Geometry: final body of the model. Coordinates: model frame, mm. Face numbers are marked on the shaded views. A direction names the side the tool comes from. Give positions to 0.01 mm unless a question says otherwise; leave off trailing zeros. Loops run counter-clockwise (first coordinate to the right, second up) from the corner with the lowest first, then second, coordinate; pieces in that order, holes last.
1. Section D-D, the plane y = -3.75. Output: boundary loops of the cut face in (x, z).
2. Material intervals for line 1 along Y through (x, z) = (12, -2.75); line 2 along Z through (x, y) = (28, -2); line 3 along Z through (x, y) = (35.5, 1.5), sorted ascending.
3. Section A-A, the plane z = 0. Output: boundary loops of the cut face in (x, y) (3 decimals).
4. Access query for the marked faces 1 and 2. Directions: +Z, -Z, +X, -X, +Y, -Y. A direction counts if a zero-diameter tool reaches every point of the face in a straight line with its end or side. Return the directions, or none.
5. First-contact query: P1, Ø2, axis at x = 21, z = -3.5, coming from the -Y side; P2, Ø1.5, axis at y = 3.5, z = 3.5, coming from the -X side; P3, Ø2, axis at y = -1, z = -3.5, coming from the +X side. Flat tips, straight axial feed; report the tip coordinate or a pass-through.
6. Section C-C, the plane x = 26. Output: boundary loops of the cut face in (y, z) (3 decimals).
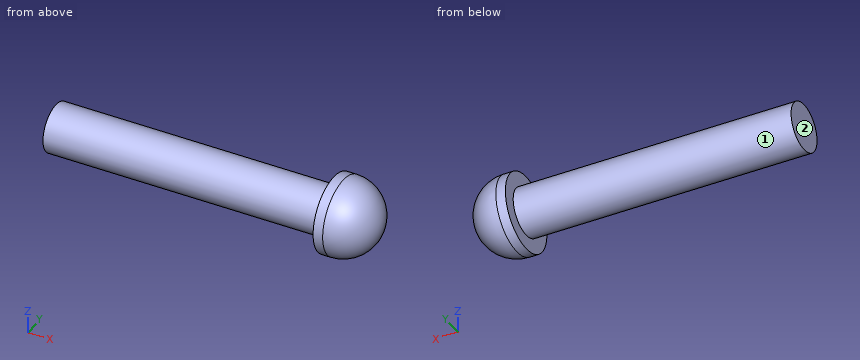
from build123d import *

# Parameters (mm, degrees)
F0_R     = 3.175
F1_DEPTH = 36.83
F2_R     = 5.08
F3_DEPTH = 6.35
F4_R     = 5.08


with BuildPart() as f1:
    # F0 (on Right) → F1 (new body)
    with BuildSketch(Plane.YZ):
        Circle(F0_R)
    extrude(amount=F1_DEPTH)

    # F2 (on face) → F3 (join)
    with BuildSketch(Plane.YZ.offset(36.83)):
        Circle(F2_R)
    extrude(amount=F3_DEPTH)

    # F4
    f4_edges = [f1.edges().sort_by_distance(p)[0] for p in [
        (43.18, -5.08, 0),
    ]]
    fillet(f4_edges, radius=F4_R)


solid = f1.part
Answers below:
1. outline: (36.83, -3.43) - (38.1, -3.43) arc R3.43 ccw to (38.1, 3.43) - (36.83, 3.43) - close
2. line 1: y = -1.59 to 1.59
2. line 2: z = -2.47 to 2.47
2. line 3: z = -2.8 to 2.8
3. outline: (0, -3.175) - (36.83, -3.175) - (36.83, -5.08) - (38.1, -5.08) arc R5.08 ccw to (38.1, 5.08) - (36.83, 5.08) - (36.83, 3.175) - (0, 3.175) - close
4. face 1: -X
4. face 2: +Z, -Z, -X, +Y, -Y
5. P1: stops at y = -1.96
5. P2: stops at x = 36.83
5. P3: stops at x = 42.44
6. outline: circle Ø6.35 at (0, 0)
